Design review of the part built by this model. Coordinates are the model's own, in mm. Coordinates: 2 decimals unless noted, no trailing zeros. Write each loop counter-clockwise with the first axis right and the second up, starting at its lowest first coordinate (ties: lowest second). Pieces come first, ordered by that corner, then holes. Notation, with made-up numbers: M 32.5,70.5 L 88.5,70.5 A8 ccw 88.5,78.5 Z; hole C 1.25,74.25 d2. An arc over 180 degrees is marked long. Return JSON: item names as keys, results as strings. Group by question number.
```python
from build123d import *

# Parameters (mm, degrees)
SKETCH1_R           = 1.55
BOSS_EXTRUDE1_DEPTH = 3


with BuildPart() as part:
    # Sketch1 → Boss-Extrude1 (new body)
    with BuildSketch(Plane(origin=(0, 0, 0), x_dir=(1, 0, 0), z_dir=(0, 1, 0))):
        Polygon((-34, 23), (34, 23), (34, 18), (37, 18), (37, 12), (34, 12), (34, -12), (37, -12), (37, -18), (34, -18), (34, -23), (-34, -23), (-34, -18), (-37, -18), (-37, -12), (-34, -12), (-34, 12), (-37, 12), (-37, 18), (-34, 18), align=None)
        with Locations(Location((19, 0, 0), (0, 0, 270))):
            Circle(SKETCH1_R, mode=Mode.SUBTRACT)
        with Locations(Location((-19, 0, 0), (0, 0, 90))):
            Circle(SKETCH1_R, mode=Mode.SUBTRACT)
    extrude(amount=BOSS_EXTRUDE1_DEPTH)


solid = part.part
```
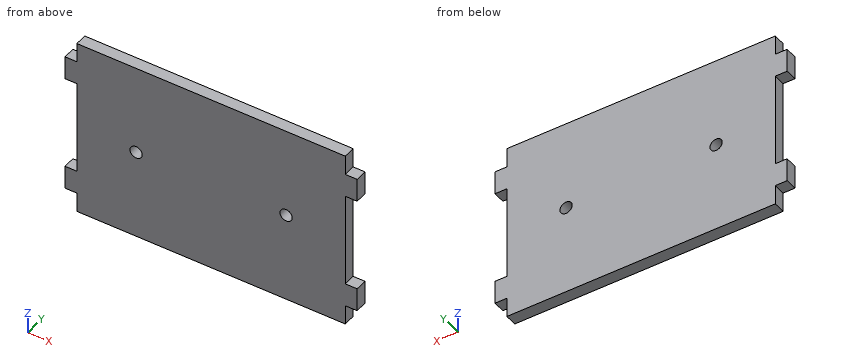
Item 1: Add section B-B (x = -19). Write out the cut boundary in (y, z), plus the area to 3 significant figures.
Item 2: Add section D-D (z = -7.5). Write out the cut boundary in (x, y).
Item 3: Add section C-C (y = 1.5). Write out the cut boundary in (x, z), plus the area to 3 significant figures.
Item 4: Add section A-A (z = 0). Write out the cut boundary in (x, y).
Item 5: For line 1 (X direction, y = 1.45, z = 0); line 2 (Z direction, x = -19, y = 2.05); line 3 (X direction, y = 2.2, z = -2), list the stretches that pass through material, from the lowest coordinate up.
Item 6: For pin 1 (0.9 mm diameter, centred on x = -35.5, y = 2, fed in from +Z); pin 2 (1.5 mm diameter, centred on x = 35, y = 1, fed in from -Z); pin 3 (1 mm diameter, centred on y = 1, z = 0.5, fed in from +X), all flat-tipped, find the tip position at first contact; note any pin that passes through.
Geometry check:
{
 "1": {"outline": "M 0,-23 L 3,-23 L 3,-1.55 L 0,-1.55 Z; M 0,1.55 L 3,1.55 L 3,23 L 0,23 Z", "area": "129 mm^2"},
 "2": {"outline": "M -34,0 L 34,0 L 34,3 L -34,3 Z"},
 "3": {"outline": "M -37,-18 L -34,-18 L -34,-23 L 34,-23 L 34,-18 L 37,-18 L 37,-12 L 34,-12 L 34,12 L 37,12 L 37,18 L 34,18 L 34,23 L -34,23 L -34,18 L -37,18 L -37,12 L -34,12 L -34,-12 L -37,-12 Z; hole C -19,0 d3.1; hole C 19,0 d3.1", "area": "3,180 mm^2"},
 "4": {"outline": "M -34,0 L -20.55,0 L -20.55,3 L -34,3 Z; M -17.45,0 L 17.45,0 L 17.45,3 L -17.45,3 Z; M 20.55,0 L 34,0 L 34,3 L 20.55,3 Z"},
 "5": {"line 1": "-34 to -20.55, -17.45 to 17.45, 20.55 to 34", "line 2": "-23 to -1.55, 1.55 to 23", "line 3": "-34 to 34"},
 "6": {"pin 1": "z = 18", "pin 2": "z = -18", "pin 3": "x = 34"}
}
